Design review of the part built by this model. Coordinates are the model's own, in mm. Face numbers are marked on the shaded views. Coordinates: 2 decimals unless noted, no trailing zeros. Loops run counter-clockwise (first coordinate to the right, second up) from the corner with the lowest first, then second, coordinate; pieces in that order, holes last. Notation, with made-up numbers: M 57,45.25 L 93,45.25 A18 cw 93,49.25 Z; hole C 89,62 d4. An arc over 180 degrees is marked long. Put each result on its own line as item: value. Start each with the question number.
(1) Clearance check with flat-ended pins moving along their axes: pin 1 (1.5 mm diameter, centred on x = 2, z = 1, fed in from -Y); pin 2 (1 mm diameter, centred on y = 1.5, z = 1.5, fed in from -X); pin 3 (1.5 mm diameter, centred on x = 1, z = 1.5, fed in from -Y). State where each tip first meets the part, or that it passes through.
(2) The part is to be moulded in two halves that separate along Y. For the marked faces 1, 2 and 3, say which applies: +Y half, -Y half, draft (parallel to the pull), parting line (faces both ways), or undercut.
(3) Take a section at C-C, the plane z = 0.9. Give the boundary of the cut face in (x, y).
(4) For probe 1 along Y at (x, z) = (-0.05, 2.4); probe 2 along Y at (x, z) = (-1.15, 0.45); probe 3 along X at (y, z) = (-1.05, 2.65), list the stretches that pass through material, from the lowest coordinate up. Write a range as [from, to].
(5) Take a section at A-A, the plane x = 0. Give the boundary of the cut face in (y, z).
(6) Take a section at D-D, the plane x = -0.65. Give the boundary of the cut face in (y, z).
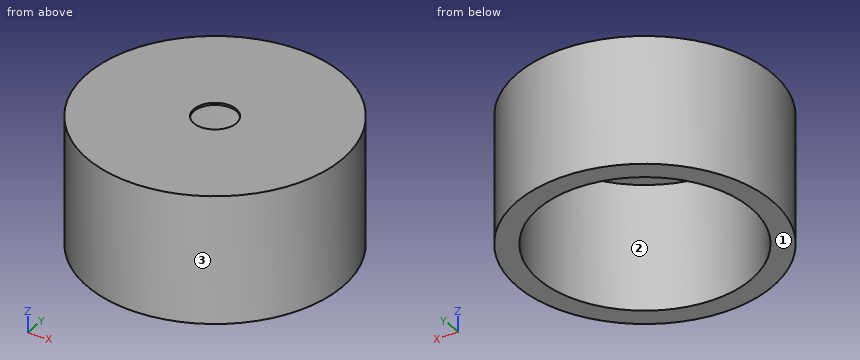
```python
from build123d import *

# Parameters (mm, degrees)
SKETCH1_R           = 3
BOSS_EXTRUDE2_DEPTH = 3
SKETCH2_R           = 2.5
CUT_EXTRUDE2_DEPTH  = 2.95
SKETCH3_R           = 0.5
CUT_EXTRUDE3_DEPTH  = 3


with BuildPart() as part:
    # Sketch1 → Boss-Extrude2 (new body)
    with BuildSketch(Plane.XY):
        Circle(SKETCH1_R)
    extrude(amount=BOSS_EXTRUDE2_DEPTH)

    # Sketch2 → Cut-Extrude2 (cut)
    with BuildSketch(Plane(origin=(0, 0, 0), x_dir=(-1, 0, 0), z_dir=(0, 0, -1))):
        Circle(SKETCH2_R)
    extrude(amount=-CUT_EXTRUDE2_DEPTH, mode=Mode.SUBTRACT)

    # Sketch3 → Cut-Extrude3 (cut)
    with BuildSketch(Plane.XY.offset(3)):
        Circle(SKETCH3_R)
    extrude(amount=-CUT_EXTRUDE3_DEPTH, mode=Mode.SUBTRACT)


solid = part.part
```
Computed values:
1. pin 1: stops at y = -2.73
1. pin 2: stops at x = -2.83
1. pin 3: stops at y = -2.99
2. face 1: draft
2. face 2: undercut
2. face 3: parting line
3. outline: C 0,0 d6; hole C 0,0 d5
4. probe 1: y = [-3, -2.5], [2.5, 3]
4. probe 2: y = [-2.77, -2.22], [2.22, 2.77]
4. probe 3: x = [-2.81, -2.27], [2.27, 2.81]
5. outline: M -3,0 L -2.5,0 L -2.5,2.95 L -0.5,2.95 L -0.5,3 L -3,3 Z; M 0.5,2.95 L 2.5,2.95 L 2.5,0 L 3,0 L 3,3 L 0.5,3 Z
6. outline: M -2.93,0 L -2.41,0 L -2.41,2.95 L 2.41,2.95 L 2.41,0 L 2.93,0 L 2.93,3 L -2.93,3 Z
